Check sheet for the modelled part. Datum: model origin and axes. Units: mm. Round coordinates to 2 decimals unless told otherwise and drop trailing zeros. Write each loop counter-clockwise with the first axis right and the second up, starting at its lowest first coordinate (ties: lowest second). Pieces come first, ordered by that corner, then holes. Notation, with made-up numbers: M 84,-15 L 142,-15 A17 ccw 142,-4 Z; hole C 1.5,28.25 d2. An arc over 180 degrees is marked long. Put each result on its own line as item: value.
```python
from build123d import *

# Parameters (mm, degrees)
SKETCH1_R           = 38.5
BOSS_EXTRUDE1_DEPTH = 10
SKETCH2_R           = 38.5
BOSS_EXTRUDE2_DEPTH = 10
BOSS_EXTRUDE3_DEPTH = 140
CUT_EXTRUDE1_REACH  = 152
SKETCH4_W           = 10
SKETCH4_H           = 10


with BuildPart() as part:
    # Sketch1 → Boss-Extrude1 (new body)
    with BuildSketch(Plane(origin=(0, 0, 0), x_dir=(1, 0, 0), z_dir=(0, 1, 0))):
        Circle(SKETCH1_R)
    extrude(amount=BOSS_EXTRUDE1_DEPTH)



with BuildPart() as body_2:
    # Sketch2 → Boss-Extrude2 (new body)
    with BuildSketch(Plane(origin=(0, 150, 0), x_dir=(1, 0, 0), z_dir=(0, 1, 0))):
        Circle(SKETCH2_R)
    extrude(amount=-BOSS_EXTRUDE2_DEPTH)


with BuildPart() as part_1:
    add(part.part)

    add(body_2.part)  # Boss-Extrude3 merges body 2
    # Sketch3 → Boss-Extrude3 (add)
    with BuildSketch(Plane(origin=(0, 10, 0), x_dir=(1, 0, 0), z_dir=(0, 1, 0))):
        with BuildLine():
            Line((38.173943993, 5), (-38.173943993, 5))
            ThreePointArc((-38.173943993, 5), (-38.5, 0), (-38.173943993, -5))
            Line((-38.173943993, -5), (38.173943993, -5))
            ThreePointArc((38.173943993, -5), (38.5, 0), (38.173943993, 5))
        make_face()
    extrude(amount=BOSS_EXTRUDE3_DEPTH)

    # Sketch4 → Cut-Extrude1 (cut, up to next)
    with BuildSketch(Plane(origin=(0, 150, 0), x_dir=(1, 0, 0), z_dir=(0, 1, 0)), mode=Mode.PRIVATE) as cut_extrude1_sk1:
        with Locations((0, 38.5)):
            Rectangle(SKETCH4_W, SKETCH4_H)
    cut_extrude1_tool1 = extrude(cut_extrude1_sk1.sketch, amount=-CUT_EXTRUDE1_REACH, mode=Mode.PRIVATE) & part_1.part
    add(cut_extrude1_tool1.solids().sort_by_distance((0, 150, -38.5))[0], mode=Mode.SUBTRACT)
    # Sketch4 → Cut-Extrude1 (cut, up to next)
    with BuildSketch(Plane(origin=(0, 150, 0), x_dir=(1, 0, 0), z_dir=(0, 1, 0)), mode=Mode.PRIVATE) as cut_extrude1_sk2:
        with Locations((0, -38.5)):
            Rectangle(SKETCH4_W, SKETCH4_H)
    cut_extrude1_tool2 = extrude(cut_extrude1_sk2.sketch, amount=-CUT_EXTRUDE1_REACH, mode=Mode.PRIVATE) & part_1.part
    add(cut_extrude1_tool2.solids().sort_by_distance((0, 150, 38.5))[0], mode=Mode.SUBTRACT)


solid = part_1.part
```
1. Cross-section at C-C (z = -13). Enter the section's corners in (x, y).
Computed values:
outline: M -36.24,0 L 36.24,0 L 36.24,10 L -36.24,10 Z; M -36.24,140 L 36.24,140 L 36.24,150 L -36.24,150 Z
2. Depth check by flat-ended pin: pin 1 Ø8 at (x, y) = (0.5, 145.5) entering from -Z; pin 2 Ø10 at (x, y) = (1, 39) entering from -Z; pin 3 Ø2 at (x, y) = (-29.5, 92) entering from +Z. Enter the tip coordinate at first touch or a pass-through.
Computed values:
pin 1: stops at z = -33.5
pin 2: stops at z = -5
pin 3: stops at z = 5
3. Cross-section at A-A (z = -27). Enter the section's corners in (x, y).
Computed values:
outline: M -27.45,0 L 27.45,0 L 27.45,10 L -27.45,10 Z; M -27.45,140 L 27.45,140 L 27.45,150 L -27.45,150 Z
4. Scan lines: probe 1 along Y at (x, z) = (-5, 11); probe 2 along Z at (x, y) = (10, 34); probe 3 along X at (y, z) = (126, 4.5). Record each from-to range of solid material in increasing order.
Computed values:
probe 1: y = 0 to 10, 140 to 150
probe 2: z = -5 to 5
probe 3: x = -38.24 to 38.24
5. Cross-section at D-D (y = 60.5). Enter the section's corners in (x, z), then the cut area to 3 significant figures.
Computed values:
outline: M -38.17,-5 L 38.17,-5 A38.5 ccw 38.17,5 L -38.17,5 A38.5 ccw Z
area: 768 mm2
6. Cross-section at B-B (x = 0). Enter the section's corners in (y, z).
Computed values:
outline: M 0,-38.5 L 10,-38.5 L 10,-5 L 140,-5 L 140,-33.5 L 150,-33.5 L 150,33.5 L 140,33.5 L 140,5 L 10,5 L 10,38.5 L 0,38.5 Z
7. Release check for a two-part mould opening along X. For faces 1 (the flat face through (-1, 74, 5)), 2 (the flat face through (0, 145, -33.5)) record: +X half, -X half, draft (parallel to the pull), parting line (faces both ways), or undercut.
Computed values:
face 1: draft
face 2: undercut
